The listing builds one solid part. Answer for the finished solid, in the listing's coordinates (mm). Face numbers are marked on the shaded views. A direction names the side the tool comes from. Coordinates: 2 decimals unless noted, no trailing zeros. Order: outer loops, then holes, each group sorted by start corner. A loop starts at its lowest first (then second) coordinate and runs counter-clockwise, first axis right, second up. Notation, with made-up numbers: (-35.75, -34.75) -> (-3.75, -34.75) arc R21 cw to (-3.75, -19.75) -> close; hole circle Ø7 at (74, 22). An arc over 180 degrees is marked (long way). Return JSON: item names as keys, results as strings.
```python
from build123d import *

# Parameters (mm, degrees)
CROQUIS1_W                 = 20.2
CROQUIS1_H                 = 15.83
SALIENTE_EXTRUIR1_DEPTH    = 31.6
CORTAR_EXTRUIR4_DEPTH      = 31.6
CORTAR_EXTRUIR5_DEPTH      = 35.649242416
CORTAR_EXTRUIR6_DEPTH      = 35.649242416
CORTAR_EXTRUIR6_DEPTH_BACK = 35.649242416
CROQUIS5_R                 = 2.025
CROQUIS6_R                 = 1.5
CORTAR_EXTRUIR7_DEPTH      = 39.814945709
CROQUIS10_W                = 20.2
CROQUIS10_H                = 8.639055001
SALIENTE_EXTRUIR4_DEPTH    = 13.5
CORTAR_EXTRUIR8_REACH      = 50.631
CROQUIS11_R                = 1.5
REDONDEO2_START            = -1
REDONDEO2_DEPTH            = 47
REDONDEO2_START_2          = -10
REDONDEO2_2_DEPTH          = 20
REDONDEO2_START_3          = -11
REDONDEO2_3_DEPTH          = 7.490944999
REDONDEO3_R                = 6


with BuildPart() as part:
    # Croquis1 → Saliente-Extruir1 (new body)
    with BuildSketch(Plane(origin=(0, 0, 0), x_dir=(1, 0, 0), z_dir=(0, 1, 0))):
        with Locations((0, 2.085)):
            Rectangle(CROQUIS1_W, CROQUIS1_H)
    extrude(amount=SALIENTE_EXTRUIR1_DEPTH)

    # Croquis2 → Cortar-Extruir4 (cut)
    with BuildSketch(Plane.XZ):
        with BuildLine():
            Line((2.78, 2.634482871), (2.78, -2.634482871))
            ThreePointArc((2.78, -2.634482871), (-3.83, 0), (2.78, 2.634482871))
        make_face()
    extrude(amount=-CORTAR_EXTRUIR4_DEPTH, mode=Mode.SUBTRACT)

    # Croquis4 → Cortar-Extruir5 (cut, through all)
    with BuildSketch(Plane.XZ):
        with BuildLine():
            Line((-0.4, -10), (-0.4, -3.809055001))
            ThreePointArc((-0.4, -3.809055001), (0, -3.83), (0.4, -3.809055001))
            Line((0.4, -3.809055001), (0.4, -10))
            Line((0.4, -10), (-0.4, -10))
        make_face()
    extrude(amount=-CORTAR_EXTRUIR5_DEPTH, mode=Mode.SUBTRACT)

    # Croquis5 → Cortar-Extruir6 (cut, two sides: drawn at the far end of the back side and taken through both)
    with BuildSketch(Plane(origin=(0, 0, 0), x_dir=(0, 0, -1), z_dir=(1, 0, 0)).offset(-CORTAR_EXTRUIR6_DEPTH_BACK)):
        with Locations((0, 6.405)):
            Circle(CROQUIS5_R)
    extrude(amount=CORTAR_EXTRUIR6_DEPTH + CORTAR_EXTRUIR6_DEPTH_BACK, mode=Mode.SUBTRACT)

    # Croquis6 → Cortar-Extruir7 (cut, through all)
    with BuildSketch(Plane(origin=(10.1, 0, 0), x_dir=(0, 0, -1), z_dir=(1, 0, 0))):
        with Locations((6.9045275, 23.8)):
            Circle(CROQUIS6_R)
        with Locations((6.9045275, 15.8)):
            Circle(CROQUIS6_R)
        with Locations((6.9045275, 7.8)):
            Circle(CROQUIS6_R)
    extrude(amount=-CORTAR_EXTRUIR7_DEPTH, mode=Mode.SUBTRACT)

    # Croquis10 → Saliente-Extruir4 (add)
    with BuildSketch(Plane(origin=(0, 31.6, 0), x_dir=(1, 0, 0), z_dir=(0, 1, 0))):
        with Locations((0, -0.810472499)):
            Rectangle(CROQUIS10_W, CROQUIS10_H)
    extrude(amount=SALIENTE_EXTRUIR4_DEPTH)

    # Croquis11 → Cortar-Extruir8 (cut, up to next)
    with BuildSketch(Plane.XY.offset(5.13), mode=Mode.PRIVATE) as cortar_extruir8_sk1:
        with Locations((-4.57, 40.8)):
            Circle(CROQUIS11_R)
    cortar_extruir8_tool1 = extrude(cortar_extruir8_sk1.sketch, amount=-CORTAR_EXTRUIR8_REACH, mode=Mode.PRIVATE) & part.part
    # Croquis11 → Cortar-Extruir8 (cut, up to next)
    with BuildSketch(Plane.XY.offset(5.13), mode=Mode.PRIVATE) as cortar_extruir8_sk2:
        with Locations((5.53, 40.8)):
            Circle(CROQUIS11_R)
    cortar_extruir8_tool2 = extrude(cortar_extruir8_sk2.sketch, amount=-CORTAR_EXTRUIR8_REACH, mode=Mode.PRIVATE) & part.part
    add(cortar_extruir8_tool1.solids().sort_by_distance((-4.57, 40.8, 5.13))[0], mode=Mode.SUBTRACT)
    add(cortar_extruir8_tool2.solids().sort_by_distance((5.53, 40.8, 5.13))[0], mode=Mode.SUBTRACT)

    # Redondeo2: read off the stored shape, not the designer's step
    # Redondeo2 outline → Redondeo2 (cut)
    with BuildSketch(Plane(origin=(0, 0, 0), x_dir=(1, 0, 0), z_dir=(0, 1, 0)).offset(REDONDEO2_START)):
        with BuildLine():
            Line((-10.1, -5.83), (-7.6, -5.83))
            ThreePointArc((-7.6, -5.83), (-9.367766953, -5.097766953), (-10.1, -3.33))
            Line((-10.1, -3.33), (-10.1, -5.83))
        make_face()
        with BuildLine():
            ThreePointArc((7.6, 10), (9.367766953, 9.267766953), (10.1, 7.5))
            Line((10.1, 7.5), (10.1, 10))
            Line((10.1, 10), (7.6, 10))
        make_face()
        with BuildLine():
            ThreePointArc((10.1, -3.33), (9.367766953, -5.097766953), (7.6, -5.83))
            Line((7.6, -5.83), (10.1, -5.83))
            Line((10.1, -5.83), (10.1, -3.33))
        make_face()
        with BuildLine():
            Line((-10.1, 10), (-10.1, 7.5))
            ThreePointArc((-10.1, 7.5), (-9.367766953, 9.267766953), (-7.6, 10))
            Line((-7.6, 10), (-10.1, 10))
        make_face()
    extrude(amount=REDONDEO2_DEPTH, mode=Mode.SUBTRACT)

    # Redondeo2 2 outline → Redondeo2 2 (cut)
    with BuildSketch(Plane.YZ.offset(REDONDEO2_START_2)):
        with BuildLine():
            ThreePointArc((29.865064843, 5.83), (30.80047919, 5.648404624), (31.6, 5.13))
            Line((31.6, 5.13), (31.6, 5.83))
            Line((31.6, 5.83), (29.865064843, 5.83))
        make_face()
    extrude(amount=REDONDEO2_2_DEPTH, mode=Mode.SUBTRACT)

    # Redondeo2 3 outline → Redondeo2 3 (cut)
    with BuildSketch(Plane.XY.offset(REDONDEO2_START_3)):
        with BuildLine():
            Line((10.1, 31.6), (7.6, 31.6))
            ThreePointArc((7.6, 31.6), (9.367766953, 30.867766953), (10.1, 29.1))
            Line((10.1, 29.1), (10.1, 31.6))
        make_face()
        with BuildLine():
            ThreePointArc((-10.1, 29.1), (-9.367766953, 30.867766953), (-7.6, 31.6))
            Line((-7.6, 31.6), (-10.1, 31.6))
            Line((-10.1, 31.6), (-10.1, 29.1))
        make_face()
    extrude(amount=REDONDEO2_3_DEPTH, mode=Mode.SUBTRACT)

    # Redondeo3
    # the kernel refuses this fillet: 6 mm, written as the material it takes off along each edge
    with BuildSketch(Plane(origin=(-10.1, 45.1, 18.33), x_dir=(1, 0, 0), z_dir=(0, 0, -1))) as redondeo3_piece_1:
        with BuildLine():
            CenterArc((REDONDEO3_R, REDONDEO3_R), REDONDEO3_R, 180, 90)
            Line((0, REDONDEO3_R), (0, 0))
            Line((0, 0), (REDONDEO3_R, 0))
        make_face()
    extrude(amount=36.839055001, mode=Mode.SUBTRACT)
    with BuildSketch(Plane(origin=(10.1, 45.1, -18.509055001), x_dir=(0, -1, 0), z_dir=(0, 0, 1))) as redondeo3_piece_2:
        with BuildLine():
            CenterArc((REDONDEO3_R, -REDONDEO3_R), REDONDEO3_R, 90, 90)
            Line((0, -REDONDEO3_R), (0, 0))
            Line((0, 0), (REDONDEO3_R, 0))
        make_face()
    extrude(amount=36.839055001, mode=Mode.SUBTRACT)


solid = part.part
```
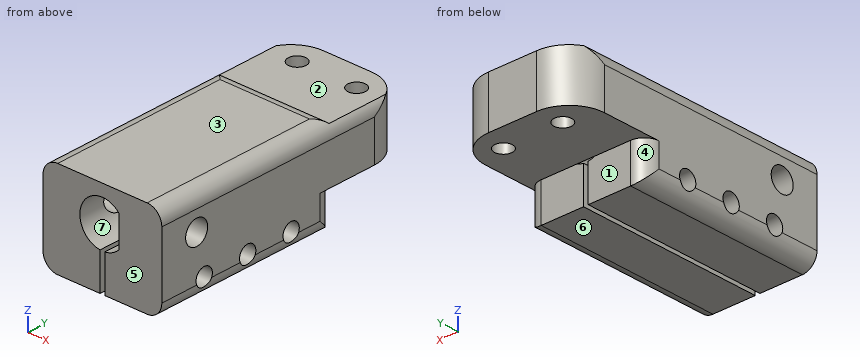
Item 1: The part is cut by section C-C on y = 23. Determine the outline of the cut face in (x, z).
Answer list:
{"outline": "(-10.1, -5.64) -> (-0.4, -5.64) -> (-0.4, -3.81) arc R3.83 cw (long way) to (2.78, 2.63) -> (2.78, -2.63) arc R3.83 cw to (0.4, -3.81) -> (0.4, -5.64) -> (10.1, -5.64) -> (10.1, 3.33) arc R2.5 ccw to (7.6, 5.83) -> (-7.6, 5.83) arc R2.5 ccw to (-10.1, 3.33) -> close; (-10.01, -8.17) arc R2.5 ccw to (-7.6, -10) -> (-0.4, -10) -> (-0.4, -8.17) -> close; (0.4, -10) -> (7.6, -10) arc R2.5 ccw to (10.01, -8.17) -> (0.4, -8.17) -> close"}
Item 2: Determine the mould class of the marked faces 5, 6 and 7 for opening direction Z: pulls with the +Z half, pulls with the -Z half, needs draft (parallel to the pull), parting line crosses it, or undercut.
Answer list:
{"face 5": "needs draft", "face 6": "pulls with the -Z half", "face 7": "undercut"}
Item 3: The part is cut by section B-B on x = -4.57. Determine the outline of the cut face in (y, z) (3 decimals), plus the area to 3 significant figures.
Answer list:
{"outline": "(0, -10) -> (31.6, -10) -> (31.6, -3.509) -> (39.3, -3.509) -> (39.3, 5.13) -> (31.6, 5.13) arc R2.5 ccw to (29.865, 5.83) -> (0, 5.83) -> close; (42.3, -3.509) -> (45.082, -3.509) -> (45.082, 5.13) -> (42.3, 5.13) -> close; hole circle Ø4.05 at (6.405, 0); hole circle Ø3 at (7.8, -6.905); hole circle Ø3 at (15.8, -6.905); hole circle Ø3 at (23.8, -6.905)", "area": "556 mm2"}
Item 4: Which of the six approach directions +Z, -Z, +X, -X, +Y, -Y give full straight-line access (tool end or side, diameter ignored) to the marked faces 1, 2, 3 and 4?
Answer list:
{"face 1": "-Z, +X, -X, +Y", "face 2": "+Z, +X, -X, +Y", "face 3": "+Z, +X, -X, +Y, -Y", "face 4": "-Z, -X, +Y"}
Item 5: The part is cut by section A-A on z = 0. Determine the outline of the cut face in (x, y).
Answer list:
{"outline": "(-10.1, 0) -> (-3.83, 0) -> (-3.83, 4.38) -> (-10.1, 4.38) -> close; (-10.1, 8.43) -> (-3.83, 8.43) -> (-3.83, 31.6) -> (2.78, 31.6) -> (2.78, 8.43) -> (10.1, 8.43) -> (10.1, 39.1) arc R6 ccw to (4.1, 45.1) -> (-4.1, 45.1) arc R6 ccw to (-10.1, 39.1) -> close; (2.78, 0) -> (10.1, 0) -> (10.1, 4.38) -> (2.78, 4.38) -> close; hole circle Ø3 at (-4.57, 40.8); hole circle Ø3 at (5.53, 40.8)"}
Item 6: Find the intervals of material crossed by probe 1 along Y at (x, z) = (5.53, -1.25); probe 2 along X at (y, z) = (28, 3.25); probe 3 along X at (y, z) = (10.5, -3.5), in increasing order.
Answer list:
{"probe 1": "0 to 4.81, 8 to 39.3, 42.3 to 44.93", "probe 2": "-10.1 to -2.03, 2.03 to 10.1", "probe 3": "-10.1 to -1.56, 1.56 to 10.1"}
Item 7: The part is cut by section D-D on y = 11. Determine the outline of the cut face in (x, z), plus the area to 3 significant figures.
Answer list:
{"outline": "(-10.1, -7.5) arc R2.5 ccw to (-7.6, -10) -> (-0.4, -10) -> (-0.4, -3.81) arc R3.83 cw (long way) to (2.78, 2.63) -> (2.78, -2.63) arc R3.83 cw to (0.4, -3.81) -> (0.4, -10) -> (7.6, -10) arc R2.5 ccw to (10.1, -7.5) -> (10.1, 3.33) arc R2.5 ccw to (7.6, 5.83) -> (-7.6, 5.83) arc R2.5 ccw to (-10.1, 3.33) -> close", "area": "267 mm2"}
Item 8: Flat-ended cylindrical pins translate along their axes: pin 1 (5 mm diameter, centred on x = -4.57, y = 40.8, fed in from +Z); pin 2 (5.5 mm diameter, centred on x = 0, z = 0, fed in from -Y); pin 3 (1.5 mm diameter, centred on x = -0.5, y = 37, fed in from -Z). Find the tip coordinate at first contact, or state that the pin passes through.
Answer list:
{"pin 1": "z = 5.13", "pin 2": "y = 31.6", "pin 3": "z = -3.51"}
